Verification items for the finished model (mm, model axes). A direction names the side the tool comes from. Give positions to 0.01 mm unless a question says otherwise; leave off trailing zeros. Write each loop counter-clockwise with the first axis right and the second up, starting at its lowest first coordinate (ties: lowest second). Pieces come first, ordered by that corner, then holes. Notation, with made-up numbers: (-27.75, 77.5) - (0.25, 77.5) arc R32 ccw to (0.25, 116.5) - close; hole circle Ø6 at (-11.75, -5). An arc over 180 degrees is marked (long way). Answer as a JSON object with one key per item and string values. Group by question number.
Item 1: Sectioned sample at B-B, the plane z = -7.25. Record the boundary of the cut face in (x, y), and give its area (3 significant figures).
Item 2: Scan lines: line 1 along Z through (x, y) = (53, 0); line 2 along Y through (x, z) = (5.25, 0) (3 decimals); line 3 along Y through (x, z) = (3.75, 0) (3 decimals). Record each from-to range of solid material in increasing order. Write a range as [from, to].
Item 3: Sectioned sample at D-D, the plane z = 1.5. Count the separate pieces of the cut face and the enclosed holes in it, and give its area (4 significant figures).
Item 4: Sectioned sample at A-A, the plane y = 0. Record the boundary of the cut face in (x, z), and give its area (3 significant figures).
Item 5: Draft check along X on faces 6 (the face through (46.146, -14.545, -12.007)), 7 (the face through (44.18, 0, -6)), 8 (the face through (3, -30, -11)). Enter one of: +X half, -X half, draft (parallel to the pull), parting line (faces both ways), or undercut.
Item 6: Go/stop test with flat-tipped pins: pin 1 (6 mm diameter, centred on y = 0, z = 0, fed in from -X); pin 2 (10 mm diameter, centred on y = 25.5, z = 0, fed in from +X); pin 3 (3 mm diameter, centred on x = 13.5, y = -29.5, fed in from -Z). Record where each tip stops, or that it passes through.
Item 7: Tool access check on faces 1 (the face through (4, -25, -3.319)), 2 (the face through (51, 0, -5.383)), 3 (the face through (57.547, -9.688, 0.668)), 4 (the face through (8, -25, -5)), 5 (the face through (28, 16.382, -1)). Record the directions out of +Z, -Z, +X, -X, +Y, -Y that give a thin tool (end or side, any length) a straight path to the whole face; none if there is none.
Item 8: Sectioned sample at C-C, the plane x = 11. Record the boundary of the cut face in (y, z), and give its area (3 significant figures).
```python
from build123d import *

# Parameters (mm, degrees)
PAD002_DEPTH    = 12.5
POCKET_DEPTH    = 23
SKETCH006_R     = 5
POCKET001_DEPTH = 13.8201293065
SKETCH007_R     = 3.175
POCKET002_DEPTH = 236.4162459853
POCKET003_DEPTH = 50
POCKET004_DEPTH = 236.4162459853
POCKET005_DEPTH = 13.8201293065
CHAMFER_SIZE    = 3
CHAMFER001_SIZE = 1


with BuildPart() as part:
    # Sketch004 → Pad002 (new body, symmetric)
    with BuildSketch(Plane.XY):
        with BuildLine():
            ThreePointArc((0, -19.5), (19.5, 0), (0, 19.5))
            Line((0, 31.5), (0, 19.5))
            Line((0, 31.5), (8, 31.5))
            Line((58, 10), (8, 31.5))
            Line((58, -10), (58, 10))
            Line((8, -31.5), (58, -10))
            Line((0, -31.5), (8, -31.5))
            Line((0, -19.5), (0, -31.5))
        make_face()
    extrude(amount=PAD002_DEPTH, both=True)

    # Sketch005 (on Face9 of Pad002) → Pocket (cut)
    with BuildSketch(Plane(origin=(0, 0, -12.5), x_dir=(1, 0, 0), z_dir=(0, 0, -1))):
        Polygon((44.1798706935, 0), (44.1798706935, 10.5), (30.5, 16.3823443982), (25.5, 16.3823443982), (25.5, 0), align=None)
    pocket = extrude(amount=-POCKET_DEPTH, mode=Mode.SUBTRACT)

    # Mirrored: Pocket across Sketch005 H_Axis
    add(pocket.mirror(Plane(origin=(0, 0, -12.5), x_dir=(0, 0, -1), z_dir=(0, -1, 0))), mode=Mode.SUBTRACT)

    # Sketch006 (on Face9 of Mirrored) → Pocket001 (cut)
    with BuildSketch(Plane.YZ.offset(58)):
        Circle(SKETCH006_R)
    extrude(amount=-POCKET001_DEPTH, mode=Mode.SUBTRACT)

    # Sketch007 (on Face1 of Pocket001) → Pocket002 (cut, through all)
    with BuildSketch(Plane(origin=(0, 0, 0), x_dir=(0, -1, 0), z_dir=(-1, 0, 0))):
        with Locations((25.5, 0)):
            Circle(SKETCH007_R)
    pocket002 = extrude(amount=-POCKET002_DEPTH, mode=Mode.SUBTRACT)

    # Mirrored001: Pocket002 across Sketch007 V_Axis
    add(pocket002.mirror(Plane(origin=(0, 0, 0), x_dir=(-1, 0, 0), z_dir=(0, -1, 0))), mode=Mode.SUBTRACT)

    # Sketch008 (on Face10 of Mirrored001) → Pocket003 (cut)
    with BuildSketch(Plane.YZ.offset(58)):
        with BuildLine():
            ThreePointArc((-19.5, 0), (-21.2573593129, 4.2426406871), (-25.5, 6))
            Line((-25.5, 6), (-31.5, 6))
            Line((-31.5, 6), (-31.5, -12.5))
            Line((-31.5, -12.5), (-19.5, -12.5))
            Line((-19.5, -12.5), (-19.5, 0))
        make_face()
    pocket003 = extrude(amount=-POCKET003_DEPTH, mode=Mode.SUBTRACT)

    # Mirrored002: Pocket003 across Sketch008 V_Axis
    add(pocket003.mirror(Plane(origin=(58, 0, 0), x_dir=(1, 0, 0), z_dir=(0, 1, 0))), mode=Mode.SUBTRACT)

    # Sketch009 (on Face1 of Mirrored002) → Pocket004 (cut, through all)
    with BuildSketch(Plane(origin=(0, 0, 0), x_dir=(0, -1, 0), z_dir=(-1, 0, 0))):
        Polygon((24.25, -2.918582704), (24.65, -3.318582704), (26.35, -3.318582704), (26.75, -2.918582704), align=None)
    pocket004 = extrude(amount=-POCKET004_DEPTH, mode=Mode.SUBTRACT)

    # Mirrored003: Pocket004 across Sketch009 V_Axis
    add(pocket004.mirror(Plane(origin=(0, 0, 0), x_dir=(-1, 0, 0), z_dir=(0, -1, 0))), mode=Mode.SUBTRACT)

    # Sketch010 (on Face16 of Mirrored003) → Pocket005 (cut)
    with BuildSketch(Plane.YZ.offset(58)):
        Polygon((-2, -4.582575695), (2, -4.582575695), (1.2, -5.382575695), (-1.2, -5.382575695), align=None)
    extrude(amount=-POCKET005_DEPTH, mode=Mode.SUBTRACT)

    # Chamfer
    chamfer_edges = [part.edges().sort_by_distance(p)[0] for p in [
        (4, -31.5, -12.5),
        (4, 31.5, -12.5),
    ]]
    chamfer(chamfer_edges, length=CHAMFER_SIZE)

    # Chamfer001
    chamfer001_edges = [part.edges().sort_by_distance(p)[0] for p in [
        (21.953488, -19.5, -12.5),
        (8, -24, -12.5),
        (8, -30, -11),
        (8, -31.5, -1.75),
        (46.953488, -14.75, -12.5),
        (58, 0, -12.5),
        (46.953488, 14.75, -12.5),
        (21.953488, 19.5, -12.5),
        (8, 24, -12.5),
        (8, 30, -11),
        (8, 31.5, -1.75),
        (58, -10, 0),
        (58, 10, 0),
    ]]
    chamfer(chamfer001_edges, length=CHAMFER001_SIZE)


solid = part.part
```
Geometry check:
{
 "1": {"outline": "(0, -31.5) - (7, -31.5) - (8, -30.5) - (8, -19.5) - (35.91, -19.5) - (57.08, -10.4) - (58, -9) - (58, 9) - (57.08, 10.4) - (35.91, 19.5) - (8, 19.5) - (8, 30.5) - (7, 31.5) - (0, 31.5) - (0, 19.5) arc R19.5 cw to (0, -19.5) - close; hole (25.5, -16.38) - (30.5, -16.38) - (44.18, -10.5) - (44.18, 10.5) - (30.5, 16.38) - (25.5, 16.38) - close", "area": "1,110 mm^2"},
 "2": {"line 1": "[-12.5, -5.38], [5, 12.5]", "line 2": "[-31.5, -28.675], [-22.325, -18.78], [18.78, 22.325], [28.675, 31.5]", "line 3": "[-31.5, -28.675], [-22.325, -19.136], [19.136, 22.325], [28.675, 31.5]"},
 "3": {"separate pieces": "3", "enclosed holes": "0", "area": "902.5 mm^2"},
 "4": {"outline": "(19.5, -12.5) - (25.5, -12.5) - (25.5, 10.5) - (44.18, 10.5) - (44.18, 5) - (58, 5) - (58, 12.5) - (19.5, 12.5) - close; (44.18, -12.5) - (57, -12.5) - (58, -11.5) - (58, -5.38) - (44.18, -5.38) - close", "area": "389 mm^2"},
 "5": {"face 6": "+X half", "face 7": "undercut", "face 8": "draft"},
 "6": {"pin 1": "x = 19.27", "pin 2": "x = 8", "pin 3": "z = 6"},
 "7": {"face 1": "+X, -X", "face 2": "+X", "face 3": "+Z, -Z, +X, -Y", "face 4": "-Z, +X, -Y", "face 5": "-Z"},
 "8": {"outline": "(-30.21, 6) - (-25.5, 6) arc R6 cw to (-19.5, 0) - (-19.5, -11.5) - (-18.5, -12.5) - (-16.1, -12.5) - (-16.1, 12.5) - (-30.21, 12.5) - close; (16.1, -12.5) - (18.5, -12.5) - (19.5, -11.5) - (19.5, 0) arc R6 cw to (25.5, 6) - (30.21, 6) - (30.21, 12.5) - (16.1, 12.5) - close", "area": "324 mm^2"}
}
